Source: CAD feature listing. Evaluate the final solid. Frame: model axes, mm. A direction names the side the tool comes from. Round coordinates to 2 decimals unless told otherwise and drop trailing zeros. Order: outer loops, then holes, each group sorted by start corner. A loop starts at its lowest first (then second) coordinate and runs counter-clockwise, first axis right, second up. Notation, with made-up numbers: (58, 74.25) - (63, 74.25) arc R27 ccw to (63, 98.25) - close; hole circle Ø2 at (10.25, 73.5). An arc over 180 degrees is marked (long way). Return JSON: item names as keys, results as strings. Group by question number.
1) Access query for faces 1 (the flat face through (12.7, 4, -12.4)), 2 (the flat face through (0, 0, 0)). Directions: +Z, -Z, +X, -X, +Y, -Y. A direction counts if a zero-diameter tool reaches every point of the face in a straight line with its end or side. Return the directions, or none.
2) Section D-D, the plane x = 44.5. Return loops of the section in (y, z), plus the area to 3 significant figures.
3) Ray query, line 1 (X direction, y = 15.5, z = -6); line 2 (X direction, y = 6.5, z = -8.5); line 3 (Y direction, x = 26, z = -3). Return the intervals inside material, ascending. Write a range as from..to.
4) Contact query for flat-ended pins moving along their axis: P1, Ø5, axis at y = -10, z = -15, coming from the +X side; P2, Ø8, axis at x = 28, z = 0.5, coming from the +Y side; P3, Ø4, axis at x = 23, y = -6.5, coming from the +Z side. Output: stop coordinate, or through.
5) Section C-C, the plane x = 10. Return loops of the section in (y, z).
6) Section A-A, the plane z = 0. Return loops of the section in (x, y).
```python
from build123d import *

# Parameters (mm, degrees)
F0_R     = 19.05
F1_DEPTH = 12.7
F2_R     = 12.573
F3_DEPTH = 50.8


with BuildPart() as f1:
    # F0 (on Right) → F1 (new body)
    with BuildSketch(Plane.YZ):
        Circle(F0_R)
    extrude(amount=F1_DEPTH)

    # F2 (on face) → F3 (join)
    with BuildSketch(Plane.YZ.offset(12.7)):
        Circle(F2_R)
    extrude(amount=F3_DEPTH)

    # F5 (on offset) → F6 (revolve, cut)
    with BuildSketch(Plane.YZ.offset(69.85)):
        with BuildLine():
            Line((0, 12.7), (0, -12.7))
            ThreePointArc((0, -12.7), (12.7, 0), (0, 12.7))
        make_face()
    revolve(axis=Axis((69.85, 0, 0), (0, 0, -1)), mode=Mode.SUBTRACT)


solid = f1.part
```
Geometry check:
{
 "1": {"face 1": "+X", "face 2": "+Z, -Z, -X, +Y, -Y"},
 "2": {"outline": "circle Ø25.15 at (0, 0)", "area": "497 mm2"},
 "3": {"line 1": "0..12.7", "line 2": "0..63.01", "line 3": "-12.21..12.21"},
 "4": {"P1": "x = 12.7", "P2": "y = 12.57", "P3": "z = 11.74"},
 "5": {"outline": "circle Ø38.1 at (0, 0)"},
 "6": {"outline": "(0, -19.05) - (12.7, -19.05) - (12.7, -12.57) - (63.5, -12.57) - (63.5, -11) arc R12.7 cw to (63.5, 11) - (63.5, 12.57) - (12.7, 12.57) - (12.7, 19.05) - (0, 19.05) - close"}
}
